Check sheet for the modelled part. Datum: model origin and axes. Units: mm. Coordinates: 2 decimals unless noted, no trailing zeros. Loops run counter-clockwise (first coordinate to the right, second up) from the corner with the lowest first, then second, coordinate; pieces in that order, holes last. Notation, with made-up numbers: (-14.5, 7) -> (4.5, 7) arc R26 cw to (4.5, 27) -> close; hole circle Ø5 at (4.5, 14.25). An arc over 180 degrees is marked (long way). Use CSV: the item, a comma, the result in double quotes. Start each with the question number.
1. Sectioned sample at A-A, the plane z = 22. Record the cut outline in (x, y), and give its area (3 significant figures).
2. Gauge pin test, flat ends, axial feed: pin 1 (10 mm diameter, centred on x = 10.5, z = 5.5, fed in from +Y); pin 2 (8 mm diameter, centred on x = 5.5, z = 14.5, fed in from +Y); pin 3 (6 mm diameter, centred on x = 37, z = 20.5, fed in from +Y). Record the tip position at first contact, or that the pin passes through.
3. Sectioned sample at B-B, the plane y = 6.75. Record the cut outline in (x, z).
4. Thickness scan on L1, parallel to Y at x = 14, z = 11; L2, parallel to X at y = 15.5, z = 2.5; L3, parallel to X at y = 11.25, z = 16. Record the ranges inside material, lowest first.
5. Sectioned sample at C-C, the plane x = 16. Record the cut outline in (y, z), and give its area (3 significant figures).
```python
from build123d import *

# Parameters (mm, degrees)
EXTRUDE1_DEPTH = 33


with BuildPart() as part:
    # Sketch1 → Extrude1 (new body)
    with BuildSketch(Plane.XY):
        with BuildLine():
            Line((0, 0), (40.5, 0))
            ThreePointArc((40.5, 0), (42.354896339, 1.252096548), (41.887283374, 3.440640427))
            Line((41.887283374, 3.440640427), (21.637283374, 22.940640427))
            ThreePointArc((21.637283374, 22.940640427), (20.25, 23.5), (18.862716626, 22.940640427))
            Line((18.862716626, 22.940640427), (-1.387283374, 3.440640427))
            ThreePointArc((-1.387283374, 3.440640427), (-1.854896339, 1.252096548), (0, 0))
        make_face()
    extrude(amount=EXTRUDE1_DEPTH)


solid = part.part
```
Completed:
1,outline,"(-1.39, 3.44) arc R2 ccw to (0, 0) -> (40.5, 0) arc R2 ccw to (41.89, 3.44) -> (21.64, 22.94) arc R2 ccw to (18.86, 22.94) -> close"
1,area,"601 mm²"
2,pin 1,"y = 19.7"
2,pin 2,"y = 13.92"
2,pin 3,"y = 11.04"
3,outline,"(2.05, 0) -> (38.45, 0) -> (38.45, 33) -> (2.05, 33) -> close"
4,L1,"0 to 18.26"
4,L2,"11.14 to 29.36"
4,L3,"6.72 to 33.78"
5,outline,"(0, 0) -> (20.18, 0) -> (20.18, 33) -> (0, 33) -> close"
5,area,"666 mm²"
